Check sheet for the modelled part. Datum: model origin and axes. Units: mm. Round coordinates to 2 decimals unless told otherwise and drop trailing zeros. Order: outer loops, then holes, each group sorted by start corner. A loop starts at its lowest first (then second) coordinate and runs counter-clockwise, first axis right, second up.
Autodesk Inventor part; units mm, degrees
ref_plane "YZ Plane" through (0, 0, 0) normal (1, 0, 0) x (0, 1, 0)
ref_plane "XZ Plane" through (0, 0, 0) normal (0, 1, 0) x (-1, 0, 0)
ref_plane "XY Plane" through (0, 0, 0) normal (0, 0, 1) x (1, 0, 0)
ref_plane "РабПлоскость1" through (0, 0, 0) normal (0, 0, 1) x (1, 0, 0)
sketch "Эскиз1" plane through (0, 0, 0) normal (0, 0, 1) x (1, 0, 0)
  circle A0 centre (-28.0013, -80.9009) radius 1.55
  circle A1 centre (-28.0013, -24.9009) radius 1.55
  circle A2 centre (27.9987, -24.9009) radius 1.55
  circle A3 centre (27.9987, -80.9009) radius 1.55
  line L0 (37.9987, -90.9009) -> (37.9987, -14.9009)
  line L1 (37.9987, -90.9009) -> (-38.0013, -90.9009)
  line L2 (-38.0013, -14.9009) -> (37.9987, -14.9009)
  line L3 (-38.0013, -14.9009) -> (-38.0013, -90.9009)
  circle A4 centre (-0.0013, -52.9009) radius 12
  circle A5 centre (-13.0013, -65.9009) radius 1.5
  circle A6 centre (-13.0013, -39.9009) radius 1.5
  circle A7 centre (12.9987, -39.9009) radius 1.5
  circle A8 centre (12.9987, -65.9009) radius 1.5
  point P0 (0, 0)
  dimension "d4" = 24
extrude "Выдавливание1" add sketch "Эскиз1" along normal blind 3
properties part number "Держатель двигателя"
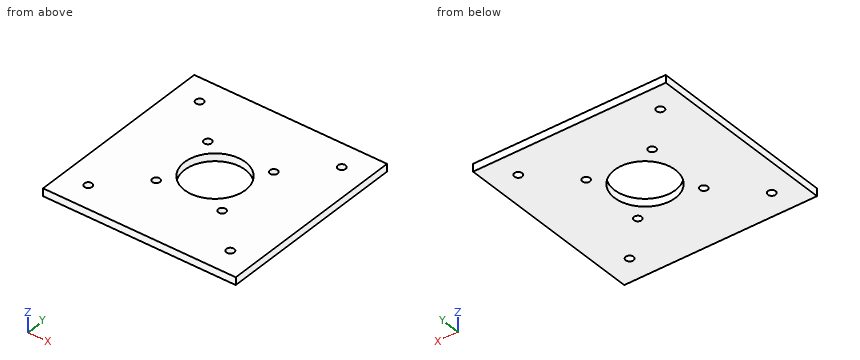
1) Sectioned sample at B-B on y = -58.5. Record the cut outline in (x, z), and give its area (3 significant figures).
2) Sectioned sample at C-C on z = 1.6. Count the separate pieces of the cut face and the enclosed holes in it, and give its area (3 significant figures).
3) Sectioned sample at A-A on x = -3. Record the cut outline in (y, z), and give its area (3 significant figures).
4) Gauge pin test, flat ends, axial feed: pin 1 (4 mm diameter, centred on x = 28, y = -80.9, fed in from -Z); pin 2 (2.5 mm diameter, centred on x = 28, y = -24.9, fed in from -Z). Record the tip position at first contact, or that the pin passes through.
5) Scan lines: line 1 (X direction, y = -66, z = 2.75); line 2 (X direction, y = -82, z = 0.95); line 3 (Y direction, x = -14, z = 1.9). Record each from-to range of solid material in increasing order.
Values found:
1. outline: (-38, 0) - (-10.61, 0) - (-10.61, 3) - (-38, 3) - close; (10.61, 0) - (38, 0) - (38, 3) - (10.61, 3) - close
1. area: 164 mm2
2. separate pieces: 1
2. enclosed holes: 9
2. area: 5,270 mm2
3. outline: (-90.9, 0) - (-64.52, 0) - (-64.52, 3) - (-90.9, 3) - close; (-41.28, 0) - (-14.9, 0) - (-14.9, 3) - (-41.28, 3) - close
3. area: 158 mm2
4. pin 1: stops at z = 0
4. pin 2: passes through
5. line 1: x = -38 to -14.5, -11.5 to 11.5, 14.5 to 38
5. line 2: x = -38 to -29.09, -26.91 to 26.91, 29.09 to 38
5. line 3: y = -90.9 to -67.02, -64.78 to -41.02, -38.78 to -14.9
